Can you work these out from the model? Positions are in its coordinate system, mm. Face numbers are marked on the shaded views. A direction names the side the tool comes from. Give positions to 0.01 mm unless a question says otherwise; leave off trailing zeros. Order: outer loops, then holes, each group sorted by start corner. A loop starts at its lowest first (then second) coordinate and runs counter-clockwise, first axis right, second up. Notation, with made-up numbers: M 30,14.25 L 63,14.25 A14 ccw 63,39.25 Z; hole C -36.75,52 d5. An arc over 180 degrees is marked long. Use one line per item in the form item = value. Start each with the question number.
1. I want a section at B-B, the plane z = 8.75. List the corners of the cut face in (x, y) for me, and give its area (3 significant figures).
2. We'd pull the mould along Z, two halves only. Please class the marked faces 3, 4 and 5: +Z half, -Z half, draft (parallel to the pull), parting line (faces both ways), or undercut.
3. Will these pins go through, and if not, where does the flat tip stop? P1, Ø4, axis at y = 5.5, z = -5, coming from the +X side; P2, Ø0.8, axis at x = -5.5, y = 2.5, coming from the -Z side; P3, Ø6, axis at x = -7, z = -1.5, coming from the +Y side.
4. I want a section at D-D, the plane x = 0. List the corners of the cut face in (y, z) for me.
5. I need wall thicknesses on L1, parallel to Y at x = 7, z = -6.5; L2, parallel to Y at x = -1.5, z = 3; L3, parallel to X at y = 1.5, z = 9.25. Which ranges of each line are inside material? Lowest first, please.
6. For the marked faces 1 and 2, which set-ups out of +Z, -Z, +X, -X, +Y, -Y let a thin tool reach every point of the face, with its end or its side?
7. I want a section at C-C, the plane x = 4.5. List the corners of the cut face in (y, z) for me.
```python
from build123d import *

# Parameters (mm, degrees)
BOSS_EXTRUDE1_DEPTH      = 1.8
SKETCH2_R                = 4
BOSS_EXTRUDE2_DEPTH      = 2.7
CUT_EXTRUDE1_DEPTH       = 2.7
BOSS_EXTRUDE3_DEPTH      = 1.5
BOSS_EXTRUDE3_DEPTH_BACK = 1.5
CUT_EXTRUDE2_START       = -1.5
SKETCH6_W                = 3
SKETCH6_H                = 2
CUT_EXTRUDE2_DEPTH       = 1.5


with BuildPart() as part:
    # Sketch1 → Boss-Extrude1 (new body)
    with BuildSketch(Plane(origin=(0, 0, 0), x_dir=(1, 0, 0), z_dir=(0, 1, 0))):
        with BuildLine():
            Line((-9.721111048, 3.25), (-9.721111048, 0))
            Line((-9.721111048, 0), (-9.721111048, -3.25))
            ThreePointArc((-9.721111048, -3.25), (-6.92820323, -4), (-7.675138086, -6.79372912))
            Line((-7.675138086, -6.79372912), (-4.860555524, -8.41872912))
            Line((-4.860555524, -8.41872912), (-2.045972962, -10.04372912))
            ThreePointArc((-2.045972962, -10.04372912), (0, -8), (2.045972962, -10.04372912))
            Line((2.045972962, -10.04372912), (4.860555524, -8.41872912))
            Line((4.860555524, -8.41872912), (7.675138086, -6.79372912))
            ThreePointArc((7.675138086, -6.79372912), (6.92820323, -4), (9.721111048, -3.25))
            Line((9.721111048, -3.25), (9.721111048, 0))
            Line((9.721111048, 0), (9.721111048, 3.25))
            ThreePointArc((9.721111048, 3.25), (6.92820323, 4), (7.675138086, 6.79372912))
            Line((7.675138086, 6.79372912), (4.860555524, 8.41872912))
            Line((4.860555524, 8.41872912), (2.045972962, 10.04372912))
            ThreePointArc((2.045972962, 10.04372912), (0, 8), (-2.045972962, 10.04372912))
            Line((-2.045972962, 10.04372912), (-4.860555524, 8.41872912))
            Line((-4.860555524, 8.41872912), (-7.675138086, 6.79372912))
            ThreePointArc((-7.675138086, 6.79372912), (-6.92820323, 4), (-9.721111048, 3.25))
        make_face()
    extrude(amount=BOSS_EXTRUDE1_DEPTH)

    # Sketch2 → Boss-Extrude2 (add)
    with BuildSketch(Plane(origin=(0, 1.8, 0), x_dir=(1, 0, 0), z_dir=(0, 1, 0))):
        with Locations(Location((0, 0, 0), (0, 0, 90))):
            Circle(SKETCH2_R)
    extrude(amount=BOSS_EXTRUDE2_DEPTH)

    # Sketch3 → Cut-Extrude1 (cut)
    with BuildSketch(Plane(origin=(0, 4.5, 0), x_dir=(1, 0, 0), z_dir=(0, 1, 0))):
        Polygon((-3.6, 5.061910399), (-3.6, -4.956827899), (3.6, -4.956827899), (3.6, 5.287050586), (4.769441753, 5.287050586), (4.769441753, -6.054386309), (-4.641273363, -6.054386309), (-4.641273363, 5.061910399), align=None)
    extrude(amount=-CUT_EXTRUDE1_DEPTH, mode=Mode.SUBTRACT)

    # Sketch4 → Revolve1 (revolve)
    with BuildSketch(Plane(origin=(0, 0, 0), x_dir=(0, 0, -1), z_dir=(1, 0, 0))):
        with BuildLine():
            Line((0, 7), (0, 4.5))
            Line((0, 4.5), (2.6, 4.5))
            ThreePointArc((2.6, 4.5), (1.80346888, 6.273607635), (0, 7))
        make_face()
    revolve(axis=Axis((0, 0, 0), (0, 1, 0)))

    # Sketch5 → Boss-Extrude3 (add, two sides: drawn at the far end of the back side and taken through both)
    with BuildSketch(Plane.XY.offset(-BOSS_EXTRUDE3_DEPTH_BACK)):
        Polygon((3.6, 3.3), (3.6, 3.1), (4.040711986, 3.1), (6.040711986, 1.8), (7.1, 1.8), (7.1, 2), (6.1, 2), (4.1, 3.3), align=None)
        Polygon((-7.1, 1.8), (-7.1, 2), (-6.1, 2), (-4.1, 3.3), (-3.6, 3.3), (-3.6, 3.1), (-4.040711986, 3.1), (-6.040711986, 1.8), align=None)
    extrude(amount=BOSS_EXTRUDE3_DEPTH + BOSS_EXTRUDE3_DEPTH_BACK)

    # Sketch6 → Cut-Extrude2 (cut)
    with BuildSketch(Plane(origin=(0, 3.3, 0), x_dir=(1, 0, 0), z_dir=(0, 1, 0)).offset(CUT_EXTRUDE2_START)):
        with Locations((-5.6, 0.5)):
            Rectangle(SKETCH6_W, SKETCH6_H)
        with Locations((5.6, -0.5)):
            Rectangle(SKETCH6_W, SKETCH6_H)
    extrude(amount=CUT_EXTRUDE2_DEPTH, mode=Mode.SUBTRACT)


solid = part.part
```
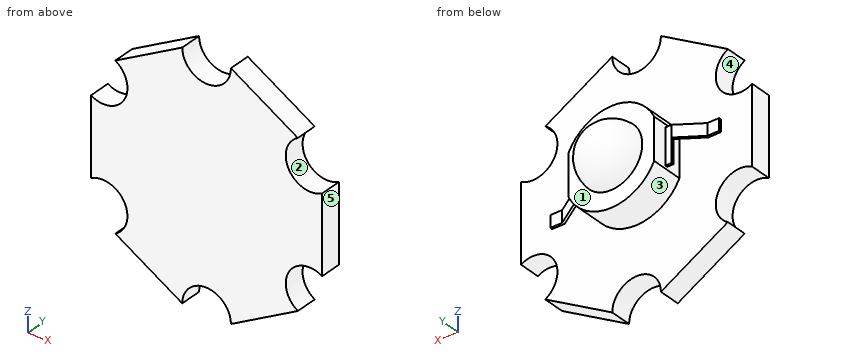
Check result:
q1.outline = M -4.29,0 L -1.58,0 L -1.58,1.8 L -4.29,1.8 Z; M 1.58,0 L 4.29,0 L 4.29,1.8 L 1.58,1.8 Z
q1.area = 9.73 mm2
q2.face_3 = -Z half
q2.face_4 = undercut
q2.face_5 = draft
q3.P1 = 2.31
q3.P2 = 0.5
q3.P3 = 3.3
q4.outline = M 0,-8 L 1.8,-8 L 1.8,-4 L 4.5,-4 L 4.5,-2.6 A2.6 ccw 4.5,2.6 L 4.5,4 L 1.8,4 L 1.8,8 L 0,8 Z
q5.L1 = 0 to 1.8
q5.L2 = 0 to 4.5
q5.L3 = -3.42 to -1.88, 1.88 to 3.42
q6.face_1 = +Y
q6.face_2 = +Y, -Y
q7.outline = M 0,-8.63 L 1.8,-8.63 L 1.8,8.63 L 0,8.63 Z; M 2.8,-1.5 L 3.04,-1.5 L 3.04,-0.5 L 2.8,-0.5 Z
